from build123d import *

# Parameters (mm, degrees)
SKETCH_3_W          = 131
SKETCH_3_H          = 80
EXTRUDE_3_DEPTH     = 5
SKETCH_4_W          = 119
SKETCH_4_H          = 80
EXTRUDE_4_DEPTH     = 6
FILLET_2_R          = 5
CHAMFER_1_SIZE      = 1
CUT_EXTRUDE_1_DEPTH = 6
FILLET_3_R          = 5
CHAMFER_2_SIZE      = 1
SKETCH_6_R          = 2.2
CUT_EXTRUDE_2_DEPTH = 11


with BuildPart() as part:
    # 草图3 → 凸台-拉伸3 (new body)
    with BuildSketch(Plane.XY):
        with Locations((0, -51.5)):
            Rectangle(SKETCH_3_W, SKETCH_3_H)
    extrude(amount=EXTRUDE_3_DEPTH)

    # 草图4 → 凸台-拉伸4 (add)
    with BuildSketch(Plane.XY.offset(5)):
        with Locations((0, -51.5)):
            Rectangle(SKETCH_4_W, SKETCH_4_H)
    extrude(amount=-EXTRUDE_4_DEPTH)

    # 圆角2
    fillet_2_edges = [part.edges().sort_by_distance(p)[0] for p in [
        (-65.5, -11.5, 2.5),
        (65.5, -11.5, 2.5),
        (65.5, -91.5, 2.5),
        (-65.5, -91.5, 2.5),
    ]]
    fillet(fillet_2_edges, radius=FILLET_2_R)

    # 倒角1
    chamfer_1_edges = [part.edges().sort_by_distance(p)[0] for p in [
        (0, -11.5, 5),
        (65.5, -51.5, 5),
        (0, -91.5, 5),
        (-65.5, -51.5, 5),
        (64.035533906, -90.035533906, 5),
        (-64.035533906, -90.035533906, 5),
        (-64.035533906, -12.964466094, 5),
        (64.035533906, -12.964466094, 5),
    ]]
    chamfer(chamfer_1_edges, length=CHAMFER_1_SIZE)

    # 草图5 → 切除-拉伸1 (cut)
    with BuildSketch(Plane.XY.offset(5)):
        Polygon((-10.644021059, -51.5), (-54.5, -28.163791023), (-54.5, -74.836208978), align=None)
        Polygon((43.855978941, -22.5), (-43.855978941, -22.5), (0, -45.836208978), align=None)
        Polygon((54.5, -28.163791023), (10.644021059, -51.5), (54.5, -74.836208978), align=None)
        Polygon((43.855978941, -80.5), (0, -57.163791023), (-43.855978941, -80.5), align=None)
    extrude(amount=-CUT_EXTRUDE_1_DEPTH, mode=Mode.SUBTRACT)

    # 圆角3
    fillet_3_edges = [part.edges().sort_by_distance(p)[0] for p in [
        (10.644021059, -51.5, 2),
        (54.5, -28.163791023, 2),
        (54.5, -74.836208978, 2),
        (-43.855978941, -22.5, 2),
        (43.855978941, -22.5, 2),
        (0, -45.836208978, 2),
        (-43.855978941, -80.5, 2),
        (0, -57.163791023, 2),
        (43.855978941, -80.5, 2),
        (-54.5, -74.836208978, 2),
        (-54.5, -28.163791023, 2),
        (-10.644021059, -51.5, 2),
    ]]
    fillet(fillet_3_edges, radius=FILLET_3_R)

    # 倒角2
    chamfer_2_edges = [part.edges().sort_by_distance(p)[0] for p in [
        (33.045284631, -39.580061586, 5),
        (54.5, -51.5, 5),
        (33.045284631, -63.419938415, 5),
        (14.256439507, -38.250213644, 5),
        (-14.256439507, -38.250213644, 5),
        (0, -22.5, 5),
        (-33.045284631, -39.580061586, 5),
        (-33.045284631, -63.419938415, 5),
        (-54.5, -51.5, 5),
        (-14.256439507, -64.749786356, 5),
        (14.256439507, -64.749786356, 5),
        (0, -80.5, 5),
        (52.074521107, -32.201893935, 5),
        (52.074521107, -70.798106066, 5),
        (16.288042118, -51.5, 5),
        (0, -45.172417956, 5),
        (-28.666695849, -26.289632976, 5),
        (28.666695849, -26.289632976, 5),
        (-16.288042118, -51.5, 5),
        (-52.074521107, -70.798106066, 5),
        (-52.074521107, -32.201893935, 5),
        (0, -57.827582045, 5),
        (28.666695849, -76.710367025, 5),
        (-28.666695849, -76.710367025, 5),
    ]]
    chamfer(chamfer_2_edges, length=CHAMFER_2_SIZE)

    # 草图6 → 切除-拉伸2 (cut)
    with BuildSketch(Plane.XY.offset(5)):
        with Locations(Location((62.5, -21.5, 0), (0, 0, 24.619977329))):
            Circle(SKETCH_6_R)
        with Locations(Location((62.5, -31.5, 0), (0, 0, 24.619977329))):
            Circle(SKETCH_6_R)
        with Locations(Location((62.5, -41.5, 0), (0, 0, 24.619977329))):
            Circle(SKETCH_6_R)
        with Locations(Location((62.5, -51.5, 0), (0, 0, 24.619977329))):
            Circle(SKETCH_6_R)
        with Locations(Location((62.5, -61.5, 0), (0, 0, 24.619977329))):
            Circle(SKETCH_6_R)
        with Locations(Location((62.5, -71.5, 0), (0, 0, 24.619977329))):
            Circle(SKETCH_6_R)
        with Locations(Location((62.5, -81.5, 0), (0, 0, 335.380022671))):
            Circle(SKETCH_6_R)
    cut_extrude_2 = extrude(amount=-CUT_EXTRUDE_2_DEPTH, mode=Mode.SUBTRACT)

    # 镜向1: 切除-拉伸2 across plane
    add(cut_extrude_2.mirror(Plane(origin=(0, 0, 0), x_dir=(0, 0, 1), z_dir=(1, 0, 0))), mode=Mode.SUBTRACT)


solid = part.part
The listing builds one solid part. Answer for the finished solid, in the listing's coordinates (mm). A direction names the side the tool comes from. Coordinates: 2 decimals unless noted, no trailing zeros. Loops run counter-clockwise (first coordinate to the right, second up) from the corner with the lowest first, then second, coordinate; pieces in that order, holes last.
1) Find section A-A on x = -12. Write down the section's boundary in (y, z), then the cut area to 3 significant figures.
2) A tool of negligible diameter and unlimited length cuts with its end or side. For faces 1 (the face through (-0.034, -45.172, 1.465)), 2 (the face through (-32.61, -39.238, 4.507)), from which of +Z, -Z, +X, -X, +Y, -Y can it reach the whole face along a straight path? Write none if from no direction.
3) Find section B-B on x = -43. Write down the section's boundary in (y, z).
4) Determine the mould class of faces 3 (the face through (-1, -51, -1)), 4 (the face through (-28.69, -76.62, 1.46)), 5 (the face through (64, -90.07, 2.03)) for opening direction Y: pulls with the +Y half, pulls with the -Y half, needs draft (parallel to the pull), parting line crosses it, or undercut.
5) Find section C-C on z = 1.75. Give the number of separate pieces and of enclosed holes in the cut face, then the cut area to 3 significant figures.
6) Flat-ended cylindrical pins translate along their axes: pin 1 Ø0.5 at (y, z) = (-47.5, -0.5) entering from -X; pin 2 Ø0.5 at (y, z) = (-53.5, -0.5) entering from +X; pin 3 Ø5 at (x, y) = (-62.5, -51.5) entering from -Z. Find the tip coordinate at first contact, or state that the pin passes through.
7) Find the intervals of material crossed by L1, parallel to X at y = -33, z = 2; L2, parallel to X at y = -79.5, z = 3; L3, parallel to X at y = -61.5, z = 1.2, in increasing order.
Values:
1. outline: (-91.5, -1) - (-80.5, -1) - (-80.5, 4) - (-81.5, 5) - (-90.5, 5) - (-91.5, 4) - close; (-63.55, -1) - (-39.45, -1) - (-39.45, 4) - (-40.58, 5) - (-62.42, 5) - (-63.55, 4) - close; (-22.5, -1) - (-11.5, -1) - (-11.5, 4) - (-12.5, 5) - (-21.5, 5) - (-22.5, 4) - close
1. area: 273 mm2
2. face 1: +Z, -Z
2. face 2: +Z
3. outline: (-91.5, -1) - (-68.72, -1) - (-68.72, 4) - (-69.85, 5) - (-90.5, 5) - (-91.5, 4) - close; (-34.28, -1) - (-11.5, -1) - (-11.5, 4) - (-12.5, 5) - (-33.15, 5) - (-34.28, 4) - close
4. face 3: needs draft
4. face 4: undercut
4. face 5: pulls with the -Y half
5. separate pieces: 1
5. enclosed holes: 18
5. area: 6,530 mm2
6. pin 1: stops at x = -59.5
6. pin 2: stops at x = 59.5
6. pin 3: stops at z = 0
7. L1: x = -65.5 to -64.11, -60.89 to -53.08, -45.41 to -24.12, 24.12 to 45.41, 53.08 to 60.89, 64.11 to 65.5
7. L2: x = -65.5 to -63.42, -61.58 to -26.82, 26.82 to 61.58, 63.42 to 65.5
7. L3: x = -65.5 to -64.7, -60.3 to -54.5, -29.44 to -8.15, 8.15 to 29.44, 54.5 to 60.3, 64.7 to 65.5
